from build123d import *

# Parameters (mm, degrees)
BOSS_EXTRUDE1_DEPTH = 9
BOSS_EXTRUDE2_DEPTH = 9
BOSS_EXTRUDE3_DEPTH = 9
FILLET1_R           = 20
SKETCH4_R           = 2.6
CUT_EXTRUDE1_DEPTH  = 184.744387669
SKETCH5_R           = 2.6
CUT_EXTRUDE2_DEPTH  = 184.744387669
SKETCH6_R           = 2.6
CUT_EXTRUDE3_DEPTH  = 189.793538025


with BuildPart() as part:
    # Sketch1 → Boss-Extrude1 (new body)
    with BuildSketch(Plane.XY):
        with BuildLine():
            Line((0, 0), (109, 0))
            Line((109, 0), (109, -39))
            ThreePointArc((109, -39), (59.502525317, -59.502525317), (39, -109))
            Line((39, -109), (0, -109))
            Line((0, -109), (0, 0))
        make_face()
    extrude(amount=BOSS_EXTRUDE1_DEPTH)

    # Sketch2 → Boss-Extrude2 (add)
    with BuildSketch(Plane(origin=(0, 0, 0), x_dir=(1, 0, 0), z_dir=(0, 1, 0))):
        with BuildLine():
            Line((0, 0), (0, 100))
            Line((0, 100), (39, 100))
            ThreePointArc((39, 100), (59.502525317, 50.502525317), (109, 30))
            Line((109, 30), (109, 0))
            Line((109, 0), (0, 0))
        make_face()
    extrude(amount=-BOSS_EXTRUDE2_DEPTH)

    # Sketch3 → Boss-Extrude3 (add)
    with BuildSketch(Plane.ZY):
        with BuildLine():
            Line((-30, -109), (0, -109))
            Line((0, -109), (0, -9))
            Line((0, -9), (-100, -9))
            Line((-100, -9), (-100, -39))
            ThreePointArc((-100, -39), (-50.502525317, -59.502525317), (-30, -109))
        make_face()
    extrude(amount=-BOSS_EXTRUDE3_DEPTH)

    # Fillet1
    fillet1_edges = [part.edges().sort_by_distance(p)[0] for p in [
        (4.5, -109, -30),
        (4.5, -39, -100),
        (39, -4.5, -100),
        (39, -109, 4.5),
        (109, -39, 4.5),
        (109, -4.5, -30),
    ]]
    fillet(fillet1_edges, radius=FILLET1_R)

    # Sketch4 → Cut-Extrude1 (cut, through all)
    with BuildSketch(Plane(origin=(0, 0, 0), x_dir=(1, 0, 0), z_dir=(0, 1, 0))):
        with Locations(Location((19, 85, 0), (0, 0, 270))):
            Circle(SKETCH4_R)
        with Locations(Location((19, 10, 0), (0, 0, 270))):
            Circle(SKETCH4_R)
        with Locations(Location((94, 10, 0), (0, 0, 270))):
            Circle(SKETCH4_R)
        with Locations(Location((49, 10, 0), (0, 0, 270))):
            Circle(SKETCH4_R)
        with Locations(Location((19, 40, 0), (0, 0, 270))):
            Circle(SKETCH4_R)
    extrude(amount=-CUT_EXTRUDE1_DEPTH, mode=Mode.SUBTRACT)

    # Sketch5 → Cut-Extrude2 (cut, through all)
    with BuildSketch(Plane.ZY):
        with Locations((-85, -19)):
            Circle(SKETCH5_R)
        with Locations((-40, -19)):
            Circle(SKETCH5_R)
        with Locations((-10, -19)):
            Circle(SKETCH5_R)
        with Locations((-10, -49)):
            Circle(SKETCH5_R)
        with Locations((-10, -94)):
            Circle(SKETCH5_R)
    extrude(amount=-CUT_EXTRUDE2_DEPTH, mode=Mode.SUBTRACT)

    # Sketch6 → Cut-Extrude3 (cut, through all)
    with BuildSketch(Plane.XY.offset(9)):
        with Locations((19, -19)):
            Circle(SKETCH6_R)
        with Locations((49, -19)):
            Circle(SKETCH6_R)
        with Locations((94, -19)):
            Circle(SKETCH6_R)
        with Locations((19, -49)):
            Circle(SKETCH6_R)
        with Locations((19, -94)):
            Circle(SKETCH6_R)
    extrude(amount=-CUT_EXTRUDE3_DEPTH, mode=Mode.SUBTRACT)


solid = part.part
Source: CAD feature listing. Evaluate the final solid. Frame: model axes, mm. A direction names the side the tool comes from. Round coordinates to 2 decimals unless told otherwise and drop trailing zeros. Loops run counter-clockwise (first coordinate to the right, second up) from the corner with the lowest first, then second, coordinate; pieces in that order, holes last. Notation, with made-up numbers: (86, -17.5) - (129, -17.5) arc R22 cw to (129, 20.5) - close; hole circle Ø4 at (86, 84.25). An arc over 180 degrees is marked (long way). Write item = value, one per line. Start each with the question number.
(1) Set-up query: faces 5 (the face through (4.44, -59.12, -50.89)), 6 (the face through (49, -47, 0)). Return all of +Z, -Z, +X, -X, +Y, -Y with unobstructed straight access to the full face (end or side cutting, diameter ignored); none if empty.
(2) Section query C-C, the plane y = -49. Output: boundary loops of the cut face in (x, z), plus the area to 3 significant figures.
(3) Section query A-A, the plane x = 19. State how many separate pieces and enclosed holes the cut face has, plus the area to 3 significant figures.
(4) Section query D-D, the plane x = 71. Output: boundary loops of the cut face in (y, z).
(5) Pin query (flat end, axial travel): pin 1 (10 mm diameter, centred on y = -30, z = -86, fed in from +X); pin 2 (4.5 mm diameter, centred on y = -94, z = -10, fed in from +X); pin 3 (8.5 mm diameter, centred on x = 19, z = -10, fed in from +Y); pin 4 (8.5 mm diameter, centred on x = 19, y = -49, fed in from -Z). Return the tip coordinate at first contact, or that it passes through.
(6) Ray query, line 1 along X through (y, z) = (-4, -10); line 2 along Y through (x, z) = (3, -10); line 3 along X through (y, z) = (-13, -10). Return the intervals inside material, ascending. Write a range as from..to.
(7) Section query B-B, the plane z = -40. Output: boundary loops of the cut face in (x, y).
(8) Pull-direction query (X, two-part tool) for faces 1 (the face through (96.578, -4.437, -10.338)), 2 (the face through (0, -42, -34)), 3 (the face through (21.578, -4.437, -10.338)), 4 (the face through (4.4, -18.9, -87.6)); classes: +X half, -X half, draft (parallel to the pull), parting line (faces both ways), or undercut.
Conclusion:
q1.face_5 = -Z, +X, -X, -Y
q1.face_6 = -Z, +X, -Y
q2.outline = (0, -63.94) - (9, -63.94) - (9, -12.6) - (0, -12.6) - close; (0, -7.4) - (9, -7.4) - (9, 0) - (16.4, 0) - (16.4, 9) - (0, 9) - close; (21.6, 0) - (72.94, 0) - (72.94, 9) - (21.6, 9) - close
q2.area = 1,140 mm2
q3.separate_pieces = 7
q3.enclosed_holes = 0
q3.area = 1,600 mm2
q4.outline = (-50.21, 0) - (-9, 0) - (-9, -41.21) - (0, -41.21) - (0, 9) - (-50.21, 9) - close
q5.pin_1 = 9
q5.pin_2 = through
q5.pin_3 = 0
q5.pin_4 = 0
q6.line_1 = 0..16.4, 21.6..46.4, 51.6..91.4, 96.6..109
q6.line_2 = -109..-96.6, -91.4..-51.6, -46.4..-21.6, -16.4..0
q6.line_3 = 0..9
q7.outline = (0, -72.94) - (9, -72.94) - (9, -21.6) - (0, -21.6) - close; (0, -16.4) - (9, -16.4) - (9, -9) - (16.4, -9) - (16.4, 0) - (0, 0) - close; (21.6, -9) - (72.94, -9) - (72.94, 0) - (21.6, 0) - close
q8.face_1 = undercut
q8.face_2 = -X half
q8.face_3 = undercut
q8.face_4 = draft
